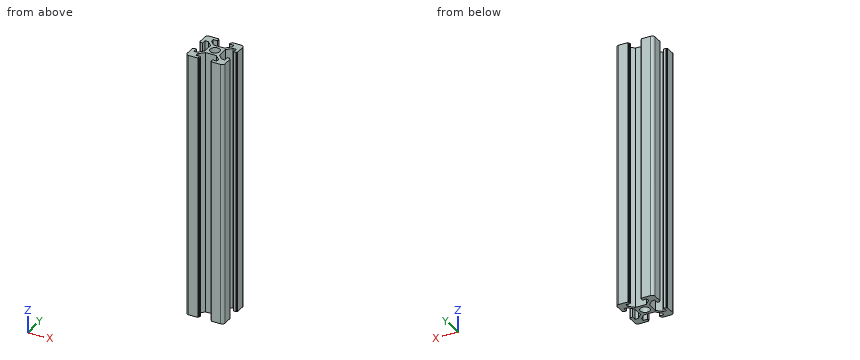
from build123d import *

# Parameters (mm, degrees)
SKETCH1_R           = 2.5
BOSS_EXTRUDE1_DEPTH = 139.7


with BuildPart() as part:
    # Sketch1 → Boss-Extrude1 (new body)
    with BuildSketch(Plane.XY):
        with BuildLine():
            Line((-10, -3.6), (-10, -8.5))
            ThreePointArc((-10, -8.5), (-9.560660172, -9.560660172), (-8.5, -10))
            Line((-8.5, -10), (-3.6, -10))
            Line((-3.6, -10), (-3.6, -9.5))
            Line((-3.6, -9.5), (-3.1, -9.5))
            Line((-3.1, -9.5), (-3.1, -8.2))
            Line((-3.1, -8.2), (-5.5, -8.2))
            Line((-5.5, -8.2), (-5.5, -6.560660172))
            Line((-5.5, -6.560660172), (-2.839339828, -3.9))
            Line((-2.839339828, -3.9), (0, -3.9))
            Line((0, -3.9), (2.839339828, -3.9))
            Line((2.839339828, -3.9), (5.5, -6.560660172))
            Line((5.5, -6.560660172), (5.5, -8.2))
            Line((5.5, -8.2), (3.1, -8.2))
            Line((3.1, -8.2), (3.1, -9.5))
            Line((3.1, -9.5), (3.6, -9.5))
            Line((3.6, -9.5), (3.6, -10))
            Line((3.6, -10), (8.5, -10))
            ThreePointArc((8.5, -10), (9.560660172, -9.560660172), (10, -8.5))
            Line((10, -8.5), (10, -3.6))
            Line((10, -3.6), (9.5, -3.6))
            Line((9.5, -3.6), (9.5, -3.1))
            Line((9.5, -3.1), (8.2, -3.1))
            Line((8.2, -3.1), (8.2, -5.5))
            Line((8.2, -5.5), (6.560660172, -5.5))
            Line((6.560660172, -5.5), (3.9, -2.839339828))
            Line((3.9, -2.839339828), (3.9, 2.839339828))
            Line((3.9, 2.839339828), (6.560660172, 5.5))
            Line((6.560660172, 5.5), (8.2, 5.5))
            Line((8.2, 5.5), (8.2, 3.1))
            Line((8.2, 3.1), (9.5, 3.1))
            Line((9.5, 3.1), (9.5, 3.6))
            Line((9.5, 3.6), (10, 3.6))
            Line((10, 3.6), (10, 8.5))
            ThreePointArc((10, 8.5), (9.560660172, 9.560660172), (8.5, 10))
            Line((8.5, 10), (3.6, 10))
            Line((3.6, 10), (3.6, 9.5))
            Line((3.6, 9.5), (3.1, 9.5))
            Line((3.1, 9.5), (3.1, 8.2))
            Line((3.1, 8.2), (5.5, 8.2))
            Line((5.5, 8.2), (5.5, 6.560660172))
            Line((5.5, 6.560660172), (2.839339828, 3.9))
            Line((2.839339828, 3.9), (0, 3.9))
            Line((0, 3.9), (-2.839339828, 3.9))
            Line((-2.839339828, 3.9), (-5.5, 6.560660172))
            Line((-5.5, 6.560660172), (-5.5, 8.2))
            Line((-5.5, 8.2), (-3.1, 8.2))
            Line((-3.1, 8.2), (-3.1, 9.5))
            Line((-3.1, 9.5), (-3.6, 9.5))
            Line((-3.6, 9.5), (-3.6, 10))
            Line((-3.6, 10), (-8.5, 10))
            ThreePointArc((-8.5, 10), (-9.560660172, 9.560660172), (-10, 8.5))
            Line((-10, 8.5), (-10, 3.6))
            Line((-10, 3.6), (-9.5, 3.6))
            Line((-9.5, 3.6), (-9.5, 3.1))
            Line((-9.5, 3.1), (-8.2, 3.1))
            Line((-8.2, 3.1), (-8.2, 5.5))
            Line((-8.2, 5.5), (-6.560660172, 5.5))
            Line((-6.560660172, 5.5), (-3.9, 2.839339828))
            Line((-3.9, 2.839339828), (-3.9, -2.839339828))
            Line((-3.9, -2.839339828), (-6.560660172, -5.5))
            Line((-6.560660172, -5.5), (-8.2, -5.5))
            Line((-8.2, -5.5), (-8.2, -3.1))
            Line((-8.2, -3.1), (-9.5, -3.1))
            Line((-9.5, -3.1), (-9.5, -3.6))
            Line((-9.5, -3.6), (-10, -3.6))
        make_face()
        Circle(SKETCH1_R, mode=Mode.SUBTRACT)
    extrude(amount=BOSS_EXTRUDE1_DEPTH)


solid = part.part
Part model, mm, in its own coordinate system. Give positions to 0.01 mm unless a question says otherwise; leave off trailing zeros. Order: outer loops, then holes, each group sorted by start corner. A loop starts at its lowest first (then second) coordinate and runs counter-clockwise, first axis right, second up. Notation, with made-up numbers: (-38.5, -35.75) -> (13.5, -35.75) arc R26 ccw to (13.5, -3.75) -> close; hole circle Ø5 at (65, 8). An arc over 180 degrees is marked (long way). Use one line per item in the form item = value.
(1) Saw through at A-A (y = 0). Write the cut outline in (x, z), then the cut area to 3 significant figures.
Solution:
outline = (-3.9, 0) -> (-2.5, 0) -> (-2.5, 139.7) -> (-3.9, 139.7) -> close; (2.5, 0) -> (3.9, 0) -> (3.9, 139.7) -> (2.5, 139.7) -> close
area = 391 mm²
(2) Drill centre lines: line 1 (Y direction, x = 0, z = 95.5); line 2 (X direction, y = 8.5, z = 16); line 3 (X direction, y = 0.25, z = 74). Where is each one in solid material? Low to high. Write a range as from..to.
Solution:
line_1 = -3.9..-2.5, 2.5..3.9
line_2 = -10..-3.1, 3.1..10
line_3 = -3.9..-2.49, 2.49..3.9
(3) Flat gauge pin, fed straight in: P1, Ø1.7, axis at y = 0.5, z = 93.5, coming from the -X side. Where does the tip first touch, or does it go through?
Solution:
P1 = -3.9
